```python
from build123d import *

# Parameters (mm, degrees)
SKETCH1_R                    = 20.5
BOSS_EXTRUDE1_DEPTH          = 5.3
SKETCH4_R                    = 8
CUT_EXTRUDE1_DEPTH           = 6.3
SKETCH6_W                    = 0.8
SKETCH6_H                    = 2.3
CUT_EXTRUDE2_DEPTH           = 10.5
CIRPATTERN3_COUNT            = 2
CIRPATTERN3_ANGLE            = 130
F_2_0_2_DIAMETER_HOLE1_D     = 2
F_2_0_2_DIAMETER_HOLE1_DEPTH = 1.9
M1_4X0_3_TAPPED_HOLE1_D      = 1.1
SKETCH41_R                   = 2.5
CUT_EXTRUDE9_DEPTH           = 3.626346
CIRPATTERN11_COUNT           = 2
CIRPATTERN11_ANGLE           = 130


with BuildPart() as part:
    # Sketch1 → Boss-Extrude1 (new body)
    with BuildSketch(Plane.XY):
        Circle(SKETCH1_R)
    extrude(amount=-BOSS_EXTRUDE1_DEPTH)

    # Sketch4 → Cut-Extrude1 (cut, through all)
    with BuildSketch(Plane.XY):
        Circle(SKETCH4_R)
    extrude(amount=-CUT_EXTRUDE1_DEPTH, mode=Mode.SUBTRACT)

    # Sketch3 → Cut-Revolve1 (revolve, cut)
    with BuildSketch(Plane(origin=(0, 0, 0), x_dir=(0, 0, -1), z_dir=(1, 0, 0))):
        Polygon((2.25, 0), (2.25, -11), (3.4, -11), (3.4, -15.6), (1, -15.6), (1, -16.35), (2.3, -16.35), (2.3, -17.5), (0, -17.5), (0, 0), align=None)
    revolve(axis=Axis((0, 0, 0), (0, 0, -1)), mode=Mode.SUBTRACT)

    # Sketch6 → Cut-Revolve2 (revolve, cut)
    with BuildSketch(Plane(origin=(0, 0, 0), x_dir=(0, 0, -1), z_dir=(1, 0, 0))):
        with Locations((0.4, -19.35)):
            Rectangle(SKETCH6_W, SKETCH6_H)
        Polygon((5.3, -16.65), (1.45, -20.5), (5.3, -20.5), align=None)
    revolve(axis=Axis((0, 0, 0), (0, 0, -1)), mode=Mode.SUBTRACT)

    # Sketch7 → Cut-Revolve3 (revolve, cut)
    with BuildSketch(Plane(origin=(0, 0, 0), x_dir=(0, 0, -1), z_dir=(1, 0, 0))):
        Polygon((1.623044738, 19.195584412), (3.602943725, 17.215685425), (3.809998961, 17.988426086), (3.885786438, 18.064213562), (2.471572875, 19.478427125), (2.395785399, 19.402639648), align=None)
    revolve(axis=Axis((0, 0, 0), (0, 0, -1)), mode=Mode.SUBTRACT)

    # Sketch12 → Cut-Extrude2 (cut)
    with BuildSketch(Plane(origin=(0, 0, 0), x_dir=(1, 0, 0), z_dir=(0, 1, 0))):
        Polygon((0, 4.814213562), (-2.564213562, 2.25), (2.564213562, 2.25), align=None)
    cut_extrude2 = extrude(amount=-CUT_EXTRUDE2_DEPTH, mode=Mode.SUBTRACT)

    # CirPattern3: Cut-Extrude2 ×2 about axis
    cirpattern3_axis = Axis((0, 0, 0), (0, 0, 1))
    for i in range(1, CIRPATTERN3_COUNT):
        add(cut_extrude2.rotate(cirpattern3_axis, i * CIRPATTERN3_ANGLE / (CIRPATTERN3_COUNT - 1)), mode=Mode.SUBTRACT)

    # 2.0 _2_ Diameter Hole1
    with Locations(Plane.XY.offset(-3.4)):
        with Locations((0, -13.5), (8.649447154, -10.365185185)):
            Hole(F_2_0_2_DIAMETER_HOLE1_D / 2, depth=F_2_0_2_DIAMETER_HOLE1_DEPTH)

    # Sketch26 → Cut-Revolve4 (revolve, cut)
    with BuildSketch(Plane(origin=(0, 0, 0), x_dir=(0, 0, -1), z_dir=(1, 0, 0))):
        Polygon((5.158578644, -16.791421356), (4.522182541, -16.155025253), (3.685666237, -16.379169121), (3.296757507, -16.768077851), (4.239339828, -17.710660172), align=None)
    revolve(axis=Axis((0, -16.508472243, -3.037151899), (0, -0.707106781, -0.707106781)), mode=Mode.SUBTRACT)

    # M1.4x0.3 Tapped Hole1 (through all)
    with Locations(Plane(origin=(0, -10.032417679, -10.032417679), x_dir=(-1, 0, 0), z_dir=(0, -0.707106781, -0.707106781))):
        with Locations((0, -9.525661966)):
            Hole(M1_4X0_3_TAPPED_HOLE1_D / 2)

    # Sketch41 → Cut-Extrude9 (cut)
    with BuildSketch(Plane(origin=(-1.547258414, 1.843950774, -2.407106781), x_dir=(0.890736799, 0.276402568, -0.360817927), z_dir=(0.454519478, -0.54167522, 0.707106781))):
        with Locations((9.491497809, 4.580281669)):
            Circle(SKETCH41_R)
    cut_extrude9 = extrude(amount=CUT_EXTRUDE9_DEPTH, mode=Mode.SUBTRACT)

    # CirPattern11: Cut-Extrude9 ×2 about axis
    cirpattern11_axis = Axis((0, 0, 0), (0, 0, -1))
    for i in range(1, CIRPATTERN11_COUNT):
        add(cut_extrude9.rotate(cirpattern11_axis, i * CIRPATTERN11_ANGLE / (CIRPATTERN11_COUNT - 1)), mode=Mode.SUBTRACT)


solid = part.part
```
For this review, take the finished solid that the model builds, in its own axes (mm). A direction names the side the tool comes from. Round coordinates to 2 decimals unless told otherwise and drop trailing zeros.
1) Insertion check: pin 1 Ø10 at (x, y) = (-13, -6.5) entering from +Z; pin 2 Ø19.5 at (x, y) = (-5.5, -3.5) entering from +Z; pin 3 Ø10 at (x, y) = (-6.5, 7.5) entering from +Z; pin 4 Ø2 at (y, z) = (-12.5, -1.5) entering from +X. Each pin has a flat end and moves straight along its axis. Give the tip position at first contact, or say it passes through.
Answer below:
pin 1: stops at z = 0
pin 2: stops at z = -1
pin 3: stops at z = -2.25
pin 4: stops at x = 16.97
2) Mouldability with a two-part tool opening along Y and no side actions: class faces 4 (the face through (-7.5, 4.1, -2.25)), 5 (the face through (19.553, 6.158, -1.12)), 6 (the face through (-18.3, 1.6, -0.8)) as +Y half, -Y half, draft (parallel to the pull), parting line (faces both ways), or undercut.
Answer below:
face 4: undercut
face 5: parting line
face 6: draft
3) For line 1 along X through (y, z) = (-1, -2); line 2 along X through (y, z) = (-11, -4.7); line 3 along Y through (x, z) = (11, -2), list the stretches that pass through material, from the lowest coordinate up.
Answer below:
line 1: x = -19.92 to -19.27, -18.79 to -17.47, -16.32 to -15.57, 15.57 to 16.32, 17.47 to 18.79, 19.27 to 19.92
line 2: x = -13.29 to -0.04, 0.11 to 7.88, 9.42 to 13.29
line 3: y = -16.64 to -15.85, -15.27 to -13.61, -12.1 to -11.06, 11.06 to 12.1, 13.61 to 15.27, 15.85 to 16.64
4) Machinability: for faces 1 (the face through (9.65, -10.32, -4.36)), 2 (the face through (-0.57, -11.41, -4)), 3 (the face through (-0.75, 17.42, -3.66)), which of the approach directions +Z, -Z, +X, -X, +Y, -Y give a long, thin tool a straight path to every point of the face, cutting with its end or side? Answer none if there is none.
Answer below:
face 1: +Z, -Z
face 2: +Z
face 3: none
